Drawing for the job (mm, zero at the part's lowest x, y, z). A direction names the side the tool comes from. Round coordinates to 2 decimals unless told otherwise and drop trailing zeros. Loops run counter-clockwise (first coordinate to the right, second up) from the corner with the lowest first, then second, coordinate; pieces in that order, holes last. Notation, with made-up numbers: M 29.5,-6.75 L 58.5,-6.75 A28 cw 58.5,11.25 Z; hole C 62,26 d9. An arc over 180 degrees is marked long. Use a Markdown table: item, result. Add a question column.
Q1. Tool access for the marked faces 1 and 2: list every direction of +Z, -Z, +X, -X, +Y, -Y with a clear straight run to the whole face (end or side of a thin tool).
Q2. Cut at C-C (y = 8.75). Give the cut face in (x, z), plus the area to 3 significant figures.
Q3. Cut at B-B (x = 17.4). Give the cut face in (y, z), plus the area to 3 significant figures.
Q4. Cut at A-A (z = 17.4). Give the cut face in (x, y), plus the area to 3 significant figures.
Q5. Pin check, flat tips, straight feed: pin 1 (4 mm diameter, centred on x = 25.5, y = 14, fed in from +Z); pin 2 (5 mm diameter, centred on x = 25, y = 14.5, fed in from -Z); pin 3 (4.5 mm diameter, centred on x = 14.5, z = 15.5, fed in from +Y); pin 4 (2 mm diameter, centred on x = 3.5, z = 24, fed in from -Y). Stop position of each tip, or through.
Q6. Probe line 1 (X direction, y = 9.75, z = 17.4); line 2 (X direction, y = 15, z = 19). List the from-to ranges inside material, lowest first. Write a range as from..to.
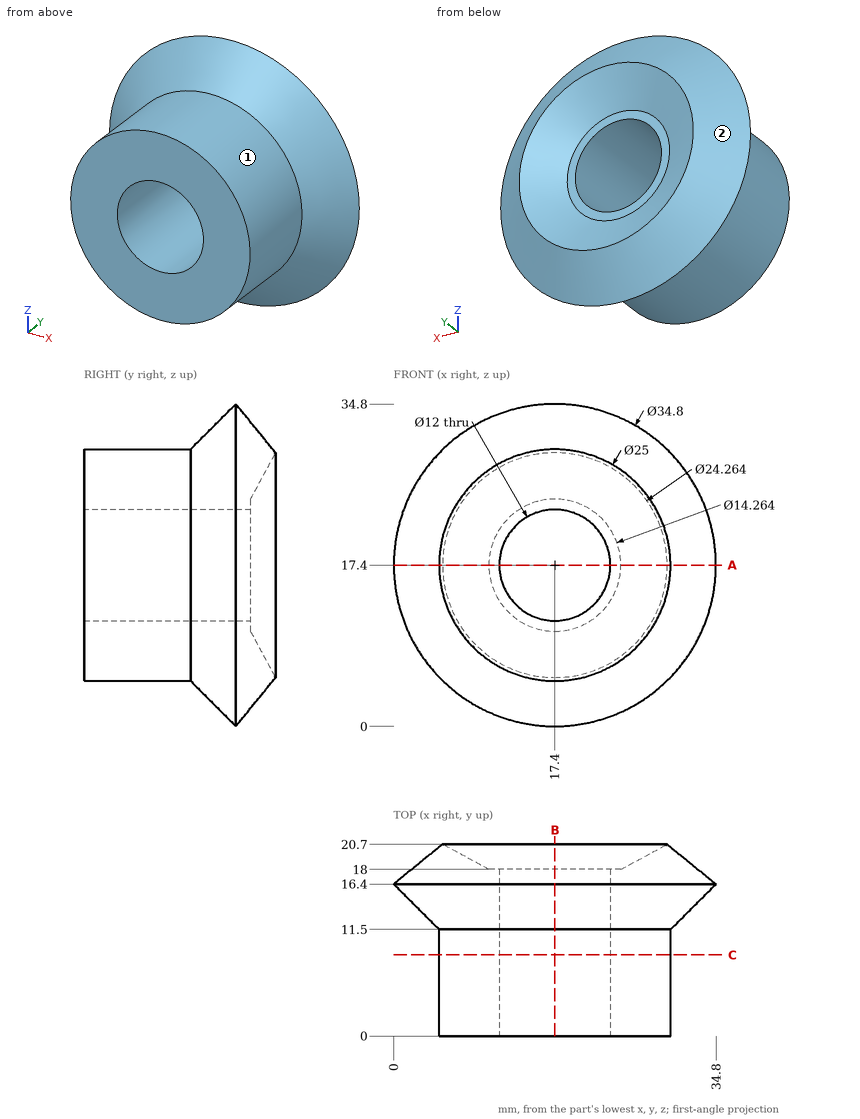
Checked values:
| question | item | result |
|---|---|---|
| 1 | face 1 | -Y |
| 1 | face 2 | +Y |
| 2 | outline | C 17.4,17.4 d25; hole C 17.4,17.4 d12 |
| 2 | area | 378 mm^2 |
| 3 | outline | M 0,4.9 L 11.5,4.9 L 16.4,0 L 20.7,5.27 L 18,10.27 L 18,11.4 L 0,11.4 Z; M 0,23.4 L 18,23.4 L 18,24.53 L 20.7,29.53 L 16.4,34.8 L 11.5,29.9 L 0,29.9 Z |
| 3 | area | 293 mm^2 |
| 4 | outline | M 0,16.4 L 4.9,11.5 L 4.9,0 L 11.4,0 L 11.4,18 L 10.27,18 L 5.27,20.7 Z; M 23.4,0 L 29.9,0 L 29.9,11.5 L 34.8,16.4 L 29.53,20.7 L 24.53,18 L 23.4,18 Z |
| 4 | area | 293 mm^2 |
| 5 | pin 1 | stops at z = 32.57 |
| 5 | pin 2 | stops at z = 1.06 |
| 5 | pin 3 | passes through |
| 5 | pin 4 | stops at y = 13.39 |
| 6 | line 1 | x = 4.9..11.4, 23.4..29.9 |
| 6 | line 2 | x = 1.48..11.62, 23.18..33.32 |
